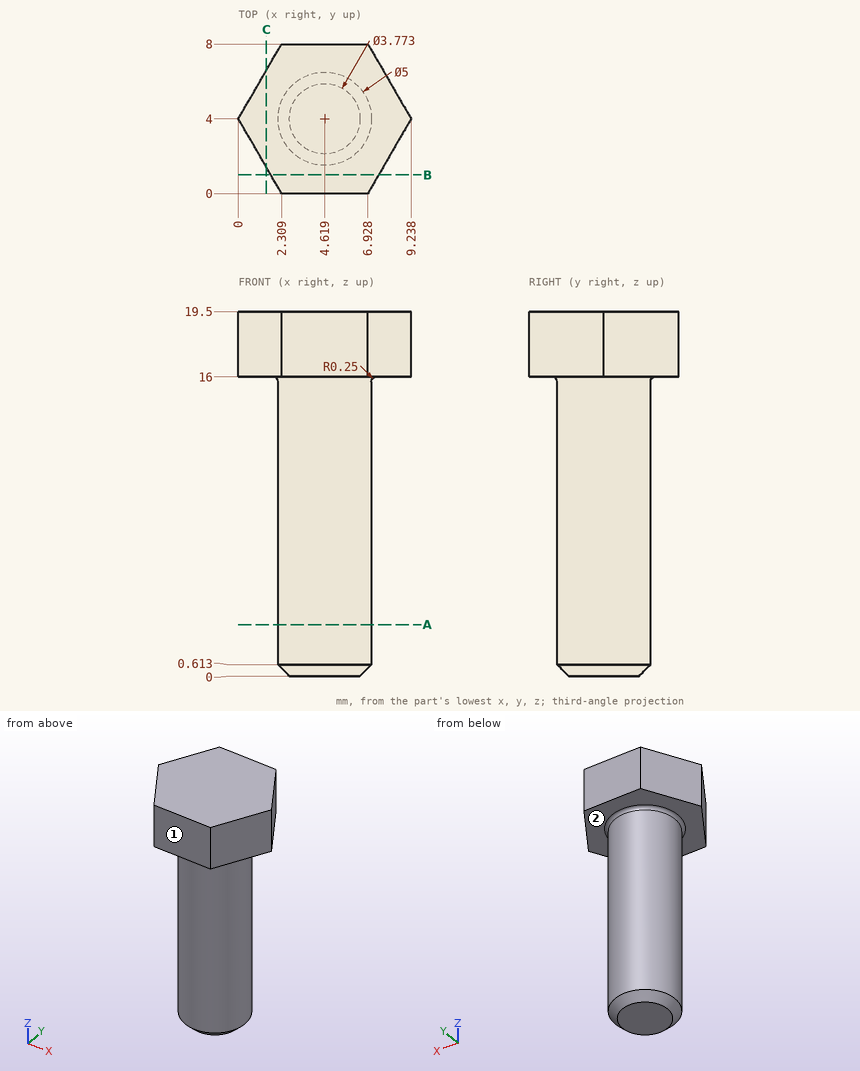
Design review of the part shown in the three views and the two pictorial views. Dimensions are in mm from the part's minimum x, y and z. A direction names the side the tool comes from. Round coordinates to 2 decimals unless told otherwise and drop trailing zeros. Write each loop counter-clockwise with the first axis right and the second up, starting at its lowest first coordinate (ties: lowest second). Pieces come first, ordered by that corner, then holes. Notation, with made-up numbers: M 42.5,42.5 L 82.5,42.5 A29 cw 82.5,64.5 Z; hole C -18,37.5 d3. An arc over 180 degrees is marked long. Use a Markdown table: item, result. Add a question column.
Q1. Insertion check: pin 1 (3 mm diameter, centred on x = 6.5, y = 2.5, fed in from -Z). The pin has a flat end and moves straight along its axis. Give the tip position at first contact, or say it passes through.
Q2. We need section C-C, the plane x = 1.5. State the section outline as (y, z) points, plus the area to 3 significant figures.
Q3. We need section B-B, the plane y = 1. State the section outline as (x, z) points (1 decimal), plus the area to 3 significant figures.
Q4. To check wall thickness, follow line 1 (Z direction, x = 1, y = 3.5); line 2 (Y direction, x = 4.5, z = 3); line 3 (X direction, y = 5, z = 14). State the ranges of each line that lie inside material, in increasing order.
Q5. We need section A-A, the plane z = 2.75. State the section outline as (x, y) points.
Q6. Machinability: for the marked faces 1 and 2, which of the approach directions +Z, -Z, +X, -X, +Y, -Y give a long, thin tool a straight path to every point of the face, cutting with its end or side? Answer none if there is none.
Findings below:
| question | item | result |
|---|---|---|
| 1 | pin 1 | stops at z = 0 |
| 2 | outline | M 1.4,16 L 6.6,16 L 6.6,19.5 L 1.4,19.5 Z |
| 2 | area | 18.2 mm² |
| 3 | outline | M 1.7,16 L 7.5,16 L 7.5,19.5 L 1.7,19.5 Z |
| 3 | area | 20.2 mm² |
| 4 | line 1 | z = 16 to 19.5 |
| 4 | line 2 | y = 1.5 to 6.5 |
| 4 | line 3 | x = 2.33 to 6.91 |
| 5 | outline | C 4.62,4 d5 |
| 6 | face 1 | +Z, -Z, +X, -X, -Y |
| 6 | face 2 | -Z |
